Build history of the part. All positions in model axes, mm. Round coordinates to 2 decimals unless told otherwise and drop trailing zeros. Order: outer loops, then holes, each group sorted by start corner. A loop starts at its lowest first (then second) coordinate and runs counter-clockwise, first axis right, second up. Notation, with made-up numbers: (77.25, 24.25) -> (124.25, 24.25) arc R15 cw to (124.25, 32.25) -> close; hole circle Ø2 at (3, 24.5). An arc over 180 degrees is marked (long way). Answer as a JSON object with one key per item and string values.
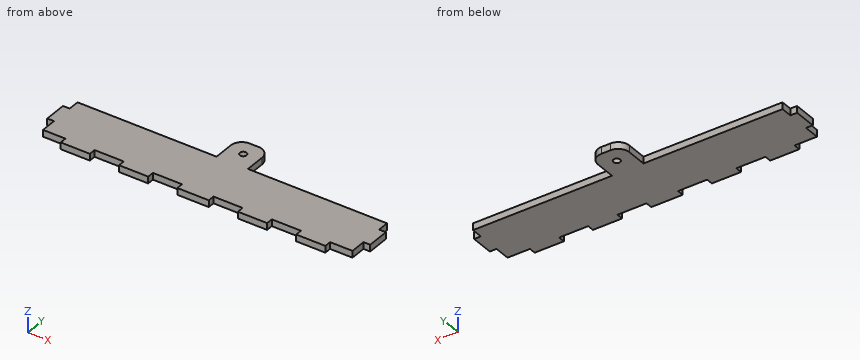
from build123d import *

# Parameters (mm, degrees)
SKETCH1_R           = 1.5
BOSS_EXTRUDE1_DEPTH = 3


with BuildPart() as part:
    # Sketch1 → Boss-Extrude1 (new body)
    with BuildSketch(Plane.XY):
        with BuildLine():
            Line((0, 17), (0, 22))
            Line((0, 22), (62, 22))
            Line((62, 22), (62, 31))
            ThreePointArc((62, 31), (63.464466094, 34.535533906), (67, 36))
            Line((67, 36), (71, 36))
            ThreePointArc((71, 36), (74.535533906, 34.535533906), (76, 31))
            Line((76, 31), (76, 22))
            Line((76, 22), (138, 22))
            Line((138, 22), (138, 17))
            Line((138, 17), (141, 17))
            Line((141, 17), (141, 7))
            Line((141, 7), (138, 7))
            Line((138, 7), (138, 0))
            Line((138, 0), (128, 0))
            Line((128, 0), (128, -3))
            Line((128, -3), (115, -3))
            Line((115, -3), (115, 0))
            Line((115, 0), (102, 0))
            Line((102, 0), (102, -3))
            Line((102, -3), (89, -3))
            Line((89, -3), (89, 0))
            Line((89, 0), (76, 0))
            Line((76, 0), (76, -3))
            Line((76, -3), (62, -3))
            Line((62, -3), (62, 0))
            Line((62, 0), (49, 0))
            Line((49, 0), (49, -3))
            Line((49, -3), (36, -3))
            Line((36, -3), (36, 0))
            Line((36, 0), (23, 0))
            Line((23, 0), (23, -3))
            Line((23, -3), (10, -3))
            Line((10, -3), (10, 0))
            Line((10, 0), (0, 0))
            Line((0, 0), (0, 7))
            Line((0, 7), (-3, 7))
            Line((-3, 7), (-3, 17))
            Line((-3, 17), (0, 17))
        make_face()
        with Locations((69, 29)):
            Circle(SKETCH1_R, mode=Mode.SUBTRACT)
    extrude(amount=BOSS_EXTRUDE1_DEPTH)


solid = part.part
1) Cut at C-C, the plane y = 23.5. Give the cut face in (x, z).
Checked values:
{"outline": "(62, 0) -> (76, 0) -> (76, 3) -> (62, 3) -> close"}
2) Probe L1, parallel to Y at x = 69, z = 0.8; L2, parallel to Y at x = 23.5, z = 2.6; L3, parallel to X at y = 24, z = 0.45. List the from-to ranges inside material, lowest first. Write a range as from..to.
Checked values:
{"L1": "y = -3..27.5, 30.5..36", "L2": "y = 0..22", "L3": "x = 62..76"}
3) Cut at B-B, the plane y = 29. Give the cut face in (x, z).
Checked values:
{"outline": "(62, 0) -> (67.5, 0) -> (67.5, 3) -> (62, 3) -> close; (70.5, 0) -> (76, 0) -> (76, 3) -> (70.5, 3) -> close"}
4) Cut at A-A, the plane x = 69. Give the cut face in (y, z), plus the area to 3 significant figures.
Checked values:
{"outline": "(-3, 0) -> (27.5, 0) -> (27.5, 3) -> (-3, 3) -> close; (30.5, 0) -> (36, 0) -> (36, 3) -> (30.5, 3) -> close", "area": "108 mm²"}
5) Flat gauge pins, fed straight in: pin 1 Ø1.5 at (x, z) = (28.5, 1) entering from -Y; pin 2 Ø0.9 at (y, z) = (2.5, 1.5) entering from -X; pin 3 Ø1.5 at (x, z) = (139.5, 1.5) entering from -Y. Where does each tip first touch, or does it go through?
Checked values:
{"pin 1": "stops at y = 0", "pin 2": "stops at x = 0", "pin 3": "stops at y = 7"}
6) Cut at D-D, the plane y = 4.5. Give the cut face in (x, z), plus the area to 3 significant figures.
Checked values:
{"outline": "(0, 0) -> (138, 0) -> (138, 3) -> (0, 3) -> close", "area": "414 mm²"}
